Here's how the part is built. I have some questions about the finished solid (model axes, mm). Coordinates: 2 decimals unless noted, no trailing zeros. Loops run counter-clockwise (first coordinate to the right, second up) from the corner with the lowest first, then second, coordinate; pieces in that order, holes last. Notation, with made-up numbers: M 37.25,66 L 93.25,66 A14 cw 93.25,78 Z; hole C -0.75,-3.75 d11. An arc over 180 degrees is marked long. Use one line per item in the form item = value. Start each with the question number.
(1) Please list where these lines run through material, in increasing order: L1, parallel to Y at x = -18, z = 1.05; L2, parallel to X at y = 156, z = 0.45.
(2) Imagine slicing it at A-A, the plane x = -27. Please give me the cut outline in (y, z).
(3) Will these pins go through, and if not, where does the flat tip stop? P1, Ø1.5, axis at x = -49, z = 2, coming from the +Y side; P2, Ø1.5, axis at x = 16.5, z = 1.5, coming from the +Y side.
(4) Imagine slicing it at B-B, the plane z = 2.25. State how many separate pieces and enclosed holes the cut face has, and give its area (3 significant figures).
(5) Imagine slicing it at C-C, the plane y = 22. Please give me the cut outline in (x, z), and give its area (3 significant figures).
```python
from build123d import *

# Parameters (mm, degrees)
SKETCH_1_W      = 20
SKETCH_1_H      = 3
SKETCH_1_H_2    = 2.958752526
EXTRUDE_1_DEPTH = 3


with BuildPart() as part:
    # 草图1 → 凸台-拉伸1 (new body)
    with BuildSketch(Plane.XY):
        Polygon((50, -50.59602649), (50, -10.59602649), (47, -10.59602649), (47, 29.40397351), (50, 29.40397351), (50, 69.40397351), (47, 69.40397351), (47, 109.40397351), (50, 109.40397351), (50, 149.40397351), (47, 149.40397351), (47, 189.40397351), (50, 189.40397351), (50, 229.40397351), (47, 229.40397351), (47, 269.40397351), (30, 269.40397351), (30, 266.40397351), (10, 266.40397351), (10, 269.40397351), (-10, 269.40397351), (-10, 266.40397351), (-30, 266.40397351), (-30, 269.40397351), (-47, 269.40397351), (-47, 229.40397351), (-50, 229.40397351), (-50, 189.40397351), (-47, 189.40397351), (-47, 149.40397351), (-50, 149.40397351), (-50, 109.40397351), (-47, 109.40397351), (-47, 69.40397351), (-50, 69.40397351), (-50, 29.40397351), (-47, 29.40397351), (-47, -10.59602649), (-50, -10.59602649), (-50, -50.59602649), align=None)
        with Locations((-20, 40.90397351)):
            Rectangle(SKETCH_1_W, SKETCH_1_H, mode=Mode.SUBTRACT)
        with Locations((-20, -9.09602649)):
            Rectangle(SKETCH_1_W, SKETCH_1_H, mode=Mode.SUBTRACT)
        with Locations((20, 40.90397351)):
            Rectangle(SKETCH_1_W, SKETCH_1_H, mode=Mode.SUBTRACT)
        with Locations((20, -9.09602649)):
            Rectangle(SKETCH_1_W, SKETCH_1_H, mode=Mode.SUBTRACT)
        with Locations((-20, 227.924597247)):
            Rectangle(SKETCH_1_W, SKETCH_1_H_2, mode=Mode.SUBTRACT)
        with Locations((20, 227.924597247)):
            Rectangle(SKETCH_1_W, SKETCH_1_H_2, mode=Mode.SUBTRACT)
    extrude(amount=EXTRUDE_1_DEPTH)


solid = part.part
```
Answer:
q1.L1 = -50.6 to -10.6, -7.6 to 39.4, 42.4 to 226.45, 229.4 to 266.4
q1.L2 = -47 to 47
q2.outline = M -50.6,0 L -10.6,0 L -10.6,3 L -50.6,3 Z; M -7.6,0 L 39.4,0 L 39.4,3 L -7.6,3 Z; M 42.4,0 L 226.45,0 L 226.45,3 L 42.4,3 Z; M 229.4,0 L 266.4,0 L 266.4,3 L 229.4,3 Z
q3.P1 = 229.4
q3.P2 = 266.4
q4.separate_pieces = 1
q4.enclosed_holes = 6
q4.area = 30,600 mm²
q5.outline = M -47,0 L 47,0 L 47,3 L -47,3 Z
q5.area = 282 mm²
